Build history of the part. All positions in model axes, mm. Face numbers are marked on the shaded views. A direction names the side the tool comes from. Round coordinates to 2 decimals unless told otherwise and drop trailing zeros. Write each loop counter-clockwise with the first axis right and the second up, starting at its lowest first coordinate (ties: lowest second). Pieces come first, ordered by that corner, then holes. Notation, with made-up numbers: M 66,47 L 94,47 A17 ccw 94,55 Z; hole C 46.5,43 d4. An arc over 180 degrees is marked long. One line per item, written item: value. Start each with the question number.
```python
from build123d import *

# Parameters (mm, degrees)
F0_R            = 40.8
F1_DEPTH        = 8
F4_R            = 32.65
F4_R_2          = 22.5
F5_DEPTH        = 2
F6_W            = 4.8
F6_H            = 38.4
F7_DEPTH        = 8.001
F9_DEPTH        = 8
F10_R           = 21
F11_DEPTH       = 8.001
F12_R           = 4
F14_D           = 3.3
F14_CBORE_D     = 6.5
F14_CBORE_DEPTH = 3
F15_SIZE        = 0.5


with BuildPart() as f1:
    # F0 (on Top) → F1 (new body)
    with BuildSketch(Plane.XY):
        Circle(F0_R)
    extrude(amount=F1_DEPTH)

    # F2 (on Right) → F3 (revolve, cut)
    with BuildSketch(Plane.YZ):
        Polygon((0, 8), (0, 0), (8.6, 0), (8.6, 6), (6.5, 6), (6.5, 8), align=None)
    revolve(axis=Axis((0, 0, 10.7360328796), (0, 0, 1)), mode=Mode.SUBTRACT)

    # F4 (on face) → F5 (cut)
    with BuildSketch(Plane.XY.offset(8)):
        Circle(F4_R)
        Circle(F4_R_2, mode=Mode.SUBTRACT)
    extrude(amount=-F5_DEPTH, mode=Mode.SUBTRACT)

    # F6 (on Top) → F7 (cut, through all)
    with BuildSketch(Plane.XY):
        with Locations((-38.4, 0)):
            Rectangle(F6_W, F6_H)
    extrude(amount=F7_DEPTH, mode=Mode.SUBTRACT)

    # F8 (on Top) → F9 (join, through all)
    with BuildSketch(Plane.XY):
        with BuildLine():
            Line((-45, 28.2782724184), (-45, -28.2782724184))
            Line((-45, -28.2782724184), (-12.6078933705, -38.8031058648))
            ThreePointArc((-12.6078933705, -38.8031058648), (-26.2059585661, -31.2711965814), (-36, -19.2))
            Line((-36, -19.2), (-36, 19.2))
            ThreePointArc((-36, 19.2), (-26.2059585661, 31.2711965814), (-12.6078933705, 38.8031058648))
            Line((-12.6078933705, 38.8031058648), (-45, 28.2782724184))
        make_face()
    extrude(amount=F9_DEPTH)

    # F10 (on face) → F11 (cut, through all)
    with BuildSketch(Plane.XY.offset(8)):
        with Locations((-56.25, 0)):
            Circle(F10_R)
    extrude(amount=-F11_DEPTH, mode=Mode.SUBTRACT)

    # F12
    f12_edges = [f1.edges().sort_by_distance(p)[0] for p in [
        (-45, -17.732386, 4),
        (-45, 17.732386, 4),
    ]]
    fillet(f12_edges, radius=F12_R)

    # F14 (through all)
    with Locations(Plane.XY.offset(8)):
        with Locations((-40.5, 24), (-40.5, -24), (37.5, 0)):
            CounterBoreHole(F14_D / 2, F14_CBORE_D / 2, F14_CBORE_DEPTH)

    # F15
    f15_edges = [f1.edges().sort_by_distance(p)[0] for p in [
        (-45, 24.044154, 0),
        (-44.588872, 18.043683, 0),
        (-28.803947, 33.540689, 0),
        (-35.25, 0, 0),
        (40.8, 0, 0),
        (-44.588872, -18.043683, 0),
        (-28.803947, -33.540689, 0),
        (-45, -24.044154, 0),
        (-42.15, -24, 0),
        (-42.15, 24, 0),
        (0, -8.6, 0),
        (35.85, 0, 0),
    ]]
    chamfer(f15_edges, length=F15_SIZE)


solid = f1.part
```
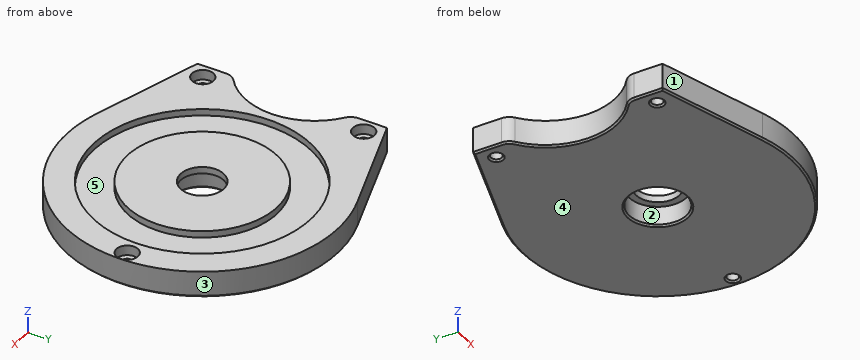
Item 1: Which spindle directions (+Z, -Z, +X, -X, +Y, -Y) get a long thin tool onto all of the face, cutting with end or side? Do the marked faces 4 and 5. Say none if no direction does.
Item 2: Cut at C-C, the plane z = 2. Write the cut outline in (x, y).
Item 3: Cut at A-A, the plane x = 0. Write the cut outline in (y, z), plus the area to 4 significant figures.
Item 4: Cut at B-B, the plane y = 0. Count the separate pieces of the cut face and the enclosed holes in it, plus the area to 3 significant figures.
Item 5: Drill centre lines: line 1 (Y direction, x = -40, z = 4.75); line 2 (Y direction, x = -40.5, z = 6); line 3 (Y direction, x = 0, z = 4.85). Where is each one in solid material? Low to high.
Item 6: Two-plate mould, pull along Y, no slides. Class the marked faces 1, 2 and 3: pulls with the +Y half, pulls with the -Y half, needs draft (parallel to the pull), parting line crosses it, or undercut.
Item 7: Drop flat-ended pins along their axis: pin 1 (2 mm diameter, centred on y = 18.5, z = 2.5, fed in from -X); pin 2 (5 mm diameter, centred on x = 37, y = -0.5, fed in from +Z); pin 3 (2 mm diameter, centred on x = 28.5, z = 5, fed in from -Y); pin 4 (3 mm diameter, centred on x = 37.5, y = 0, fed in from -Z). Give the stop position or say it passes through.
Computed values:
1. face 4: -Z, +X, -X, +Y, -Y
1. face 5: +Z
2. outline: M -45,-28.28 L -12.61,-38.8 A40.8 ccw long -12.61,38.8 L -45,28.28 L -45,19.81 A4 ccw -43.44,16.64 A21 cw -43.44,-16.64 A4 ccw -45,-19.81 Z; hole C -40.5,-24 d3.3; hole C -40.5,24 d3.3; hole C 0,0 d17.2; hole C 37.5,0 d3.3
3. outline: M -40.8,0.5 L -40.3,0 L -9.1,0 L -8.6,0.5 L -8.6,6 L -6.5,6 L -6.5,8 L -22.5,8 L -22.5,6 L -32.65,6 L -32.65,8 L -40.8,8 Z; M 6.5,6 L 8.6,6 L 8.6,0.5 L 9.1,0 L 40.3,0 L 40.8,0.5 L 40.8,8 L 32.65,8 L 32.65,6 L 22.5,6 L 22.5,8 L 6.5,8 Z
3. area: 482.5 mm2
4. separate pieces: 3
4. enclosed holes: 0
4. area: 402 mm2
5. line 1: y = -29.9 to -25.57, -22.43 to -13.3, 13.3 to 22.43, 25.57 to 29.9
5. line 2: y = -29.74 to -27.25, -20.75 to -13.89, 13.89 to 20.75, 27.25 to 29.74
5. line 3: y = -40.8 to -8.6, 8.6 to 40.8
6. face 1: pulls with the -Y half
6. face 2: undercut
6. face 3: parting line crosses it
7. pin 1: stops at x = -44.99
7. pin 2: stops at z = 5
7. pin 3: stops at y = -30.14
7. pin 4: passes through
